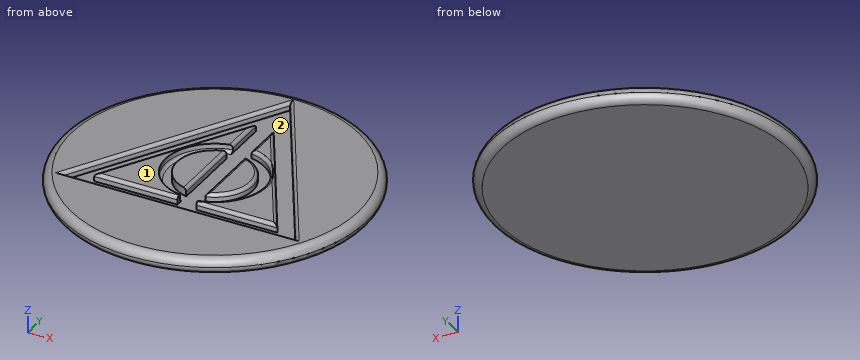
from build123d import *

# Parameters (mm, degrees)
F0_R         = 47.5
F1_DEPTH     = 5
F3_DEPTH     = 2.5
F4_R         = 15.4938561144
F4_R_2       = 11.9238234347
F5_DEPTH     = 2.5
F7_DEPTH     = 2.5
F8_R         = 2.49999
F9_T1_DEPTH  = 79.5044599257
F9_T6_ANGLE  = 178.5086872517
F9_T8_DEPTH  = 27.9406148573
F9_T10_DEPTH = 28.2323532374
F9_T12_DEPTH = 17.7111990238
F9_T14_DEPTH = 18.2220956401
F9_T16_DEPTH = 31.2335819135
F9_T18_DEPTH = 30.5369030224
F9_T20_DEPTH = 56.4226854656
F9_T22_DEPTH = 57.113596888
F9_T25_ANGLE = 172.3459061433
F9_T27_ANGLE = 174.2406786555
F9_T31_DEPTH = 79.5044599257
F9_T37_DEPTH = 79.5044599257
F9_T44_DEPTH = 79.5044599257
F9_T48_DEPTH = 79.5044599257


# Not quite as in the source:
# - a fillet or chamfer that OpenCascade refuses, or shapes differently, is made with other operations: its cross-section is extruded or revolved along the edge and cut away or added
# - a fillet or chamfer is up to 0.001 mm smaller than in the source, because OpenCascade refuses the exact size


with BuildPart() as f1:
    # F0 (on Top) → F1 (new body)
    with BuildSketch(Plane.XY):
        Circle(F0_R)
    extrude(amount=F1_DEPTH)

    # F2 (on face) → F3 (cut)
    with BuildSketch(Plane.XY.offset(5)):
        Polygon((-37.336189985, -21.3615019839), (37.1676983736, -21.6533380156), (0.1684916114, 43.0148399995), align=None)
        Polygon((-28.924478218, -16.5488310158), (0.1305310463, 33.3237484359), (28.7939471716, -16.77491742), align=None, mode=Mode.SUBTRACT)
    extrude(amount=-F3_DEPTH, mode=Mode.SUBTRACT)

    # F4 (on face) → F5 (cut)
    with BuildSketch(Plane.XY.offset(5)):
        Circle(F4_R)
        Circle(F4_R_2, mode=Mode.SUBTRACT)
    extrude(amount=-F5_DEPTH, mode=Mode.SUBTRACT)

    # F6 (on face) → F7 (cut)
    with BuildSketch(Plane.XY.offset(5)):
        with BuildLine():
            Line((3.2572400577, 27.8588049238), (0.1305310463, 33.3237484359))
            Line((0.1305310463, 33.3237484359), (-2.6910975575, 28.4804563395))
            Line((-2.6910975575, 28.4804563395), (-2.6910975575, 15.2583606993))
            ThreePointArc((-2.6910975575, 15.2583606993), (0.2884371491, 15.491171076), (3.2572400577, 15.1476059))
            Line((3.2572400577, 15.1476059), (3.2572400577, 27.8588049238))
        make_face()
        with BuildLine():
            ThreePointArc((3.2572400577, 15.1476059), (0.2884371491, 15.491171076), (-2.6910975575, 15.2583606993))
            Line((-2.6910975575, 15.2583606993), (-2.6910975575, -15.2583606993))
            ThreePointArc((-2.6910975575, -15.2583606993), (0.2884371491, -15.491171076), (3.2572400577, -15.1476059))
            Line((3.2572400577, -15.1476059), (3.2572400577, 15.1476059))
        make_face()
        with BuildLine():
            ThreePointArc((3.2572400577, -15.1476059), (0.2884371491, -15.491171076), (-2.6910975575, -15.2583606993))
            Line((-2.6910975575, -15.2583606993), (-2.6910975575, -16.6515886823))
            Line((-2.6910975575, -16.6515886823), (3.2572400577, -16.6748886641))
            Line((3.2572400577, -16.6748886641), (3.2572400577, -15.1476059))
        make_face()
    extrude(amount=-F7_DEPTH, mode=Mode.SUBTRACT)

    # F8 (radius 2.5 in the source; OpenCascade refuses exactly that, so slightly less here)
    f8_edges = [f1.edges().sort_by_distance(p)[0] for p in [
        (-47.5, 0, 5),
        (-47.5, 0, 0),
    ]]
    fillet(f8_edges, radius=F8_R)

    # F9: fillet of radius 1 on 14 edges, made by hand

    # F9_s2 → F9_t1 (join)
    with BuildSketch(Plane(origin=(-39.7519250003, 0.155710585, 0), x_dir=(0, 0, 1), z_dir=(0.9999923284, -0.0039170277, 0))):
        with BuildLine():
            ThreePointArc((3.5, 21.507584997), (2.7928932188, 21.2146917781), (2.5, 20.507584997))
            Line((2.5, 20.507584997), (2.5, 21.507584997))
            Line((2.5, 21.507584997), (3.5, 21.507584997))
        make_face()
    extrude(amount=F9_T1_DEPTH)


with BuildPart() as f9_tool4:
    # F9_s5 → F9_t6 (revolve)
    with BuildSketch(Plane(origin=(0, 0, 0), x_dir=(0, 0, 1), z_dir=(0.999915317, 0.0130137915, 0))):
        with BuildLine():
            ThreePointArc((2.5, -14.4938561144), (2.7928932188, -15.2009628956), (3.5, -15.4938561144))
            Line((3.5, -15.4938561144), (2.5, -15.4938561144))
            Line((2.5, -15.4938561144), (2.5, -14.4938561144))
        make_face()
    revolve(axis=Axis((0, 0, 2.5), (0, 0, 1)), revolution_arc=F9_T6_ANGLE)

    split(bisect_by=Plane.YZ.offset(-2.6910975575), keep=Keep.BOTTOM)


with BuildPart() as f1_1:
    add(f1.part)

    # F9_t3: union F9_tool4
    add(f9_tool4.part)

    # F9_s9 → F9_t8 (cut)
    with BuildSketch(Plane.XZ.offset(-13.9703074287)):
        with BuildLine():
            ThreePointArc((4.2572400577, 5), (3.5501332765, 4.7071067812), (3.2572400577, 4))
            Line((3.2572400577, 4), (3.2572400577, 5))
            Line((3.2572400577, 5), (4.2572400577, 5))
        make_face()
    extrude(amount=F9_T8_DEPTH, mode=Mode.SUBTRACT)

    # F9_s11 → F9_t10 (cut)
    with BuildSketch(Plane.XZ.offset(-14.1161766187)):
        with BuildLine():
            ThreePointArc((-2.6910975575, 4), (-2.9839907764, 4.7071067812), (-3.6910975575, 5))
            Line((-3.6910975575, 5), (-2.6910975575, 5))
            Line((-2.6910975575, 5), (-2.6910975575, 4))
        make_face()
    extrude(amount=F9_T10_DEPTH, mode=Mode.SUBTRACT)

    # F9_s13 → F9_t12 (cut)
    with BuildSketch(Plane.XZ.offset(-30.3588049238)):
        with BuildLine():
            ThreePointArc((4.2572400577, 5), (3.5501332765, 4.7071067812), (3.2572400577, 4))
            Line((3.2572400577, 4), (3.2572400577, 5))
            Line((3.2572400577, 5), (4.2572400577, 5))
        make_face()
    extrude(amount=F9_T12_DEPTH, mode=Mode.SUBTRACT)

    # F9_s15 → F9_t14 (cut)
    with BuildSketch(Plane.XZ.offset(-30.9804563395)):
        with BuildLine():
            ThreePointArc((-3.6910975575, 5), (-2.9839907764, 4.7071067812), (-2.6910975575, 4))
            Line((-2.6910975575, 4), (-2.6910975575, 5))
            Line((-2.6910975575, 5), (-3.6910975575, 5))
        make_face()
    extrude(amount=F9_T14_DEPTH, mode=Mode.SUBTRACT)

    # F9_s17 → F9_t16 (cut)
    with BuildSketch(Plane(origin=(-0.1258512133, 0.0004929665, 0), x_dir=(0, 0, 1), z_dir=(-0.9999923284, 0.0039170277, 0))):
        with BuildLine():
            ThreePointArc((5, -15.6620020419), (4.7071067812, -16.369108823), (4, -16.6620020419))
            Line((4, -16.6620020419), (5, -16.6620020419))
            Line((5, -16.6620020419), (5, -15.6620020419))
        make_face()
    extrude(amount=F9_T16_DEPTH, mode=Mode.SUBTRACT)

    # F9_s19 → F9_t18 (cut)
    with BuildSketch(Plane(origin=(31.3591935158, -0.1228357713, 0), x_dir=(0, 0, 1), z_dir=(-0.9999923284, 0.0039170277, 0))):
        with BuildLine():
            ThreePointArc((5, -15.6620020419), (4.7071067812, -16.369108823), (4, -16.6620020419))
            Line((4, -16.6620020419), (5, -16.6620020419))
            Line((5, -16.6620020419), (5, -15.6620020419))
        make_face()
    extrude(amount=F9_T18_DEPTH, mode=Mode.SUBTRACT)

    # F9_s21 → F9_t20 (cut)
    with BuildSketch(Plane(origin=(-12.4465088481, 21.7543326005, 0), x_dir=(0, 0, 1), z_dir=(0.4966039187, -0.8679772738, 0))):
        with BuildLine():
            ThreePointArc((4, -16.6620020419), (4.7071067812, -16.369108823), (5, -15.6620020419))
            Line((5, -15.6620020419), (5, -16.6620020419))
            Line((5, -16.6620020419), (4, -16.6620020419))
        make_face()
    extrude(amount=F9_T20_DEPTH, mode=Mode.SUBTRACT)

    # F9_s23 → F9_t22 (cut)
    with BuildSketch(Plane(origin=(-15.7859756564, -27.0964403413, 0), x_dir=(0, 0, 1), z_dir=(0.5033884097, 0.8640602462, 0))):
        with BuildLine():
            ThreePointArc((5, -15.6620020419), (4.7071067812, -16.369108823), (4, -16.6620020419))
            Line((4, -16.6620020419), (5, -16.6620020419))
            Line((5, -16.6620020419), (5, -15.6620020419))
        make_face()
    extrude(amount=F9_T22_DEPTH, mode=Mode.SUBTRACT)

    # F9_s24 → F9_t25 (revolve, cut)
    with BuildSketch(Plane(origin=(0, 0, 0), x_dir=(0, 0, 1), z_dir=(-0.997770072, 0.0667449131, 0))):
        with BuildLine():
            ThreePointArc((4, 11.9238234347), (4.7071067812, 11.6309302159), (5, 10.9238234347))
            Line((5, 10.9238234347), (5, 11.9238234347))
            Line((5, 11.9238234347), (4, 11.9238234347))
        make_face()
    revolve(axis=Axis((0, 0, 5), (0, 0, -1)), revolution_arc=F9_T25_ANGLE, mode=Mode.SUBTRACT)

    # F9_s26 → F9_t27 (revolve, cut)
    with BuildSketch(Plane(origin=(0, 0, 0), x_dir=(0, 0, 1), z_dir=(-0.9987372542, 0.0502384033, 0))):
        with BuildLine():
            ThreePointArc((5, 16.4938561144), (4.7071067812, 15.7867493333), (4, 15.4938561144))
            Line((4, 15.4938561144), (5, 15.4938561144))
            Line((5, 15.4938561144), (5, 16.4938561144))
        make_face()
    revolve(axis=Axis((0, 0, 5), (0, 0, -1)), revolution_arc=F9_T27_ANGLE, mode=Mode.SUBTRACT)


with BuildPart() as f9_tool29:
    # F9_s30 → F9_t31 (new body)
    with BuildSketch(Plane(origin=(20.0108118224, 34.3483216071, 0), x_dir=(0, 0, 1), z_dir=(-0.5033884097, -0.8640602462, 0))):
        with BuildLine():
            ThreePointArc((5, 22.507584997), (4.7071067812, 21.8004782158), (4, 21.507584997))
            Line((4, 21.507584997), (5, 21.507584997))
            Line((5, 21.507584997), (5, 22.507584997))
        make_face()
    extrude(amount=F9_T31_DEPTH)

    split(bisect_by=Plane(origin=(18.6680949925, 10.680750992, 0), x_dir=(0, 0, 1), z_dir=(-0.8679772738, -0.4966039187, 0)), keep=Keep.TOP)

    split(bisect_by=Plane(origin=(-0.0842458057, -21.5074199997, 0), x_dir=(0, 0, 1), z_dir=(0.0039170277, 0.9999923284, 0)), keep=Keep.TOP)


with BuildPart() as f1_2:
    add(f1_1.part)

    # F9_t28: cut F9_tool29
    add(f9_tool29.part, mode=Mode.SUBTRACT)


with BuildPart() as f9_tool35:
    # F9_s36 → F9_t37 (new body)
    with BuildSketch(Plane(origin=(19.7411131779, -34.5040321921, 0), x_dir=(0, 0, 1), z_dir=(-0.4966039187, 0.8679772738, 0))):
        with BuildLine():
            ThreePointArc((5, 22.507584997), (4.7071067812, 21.8004782158), (4, 21.507584997))
            Line((4, 21.507584997), (5, 21.507584997))
            Line((5, 21.507584997), (5, 22.507584997))
        make_face()
    extrude(amount=F9_T37_DEPTH)

    split(bisect_by=Plane(origin=(-18.5838491868, 10.8266690078, 0), x_dir=(0, 0, 1), z_dir=(0.8640602462, -0.5033884097, 0)), keep=Keep.TOP)

    split(bisect_by=Plane(origin=(-0.0842458057, -21.5074199997, 0), x_dir=(0, 0, 1), z_dir=(0.0039170277, 0.9999923284, 0)), keep=Keep.TOP)


with BuildPart() as f1_3:
    add(f1_2.part)

    # F9_t34: cut F9_tool35
    add(f9_tool35.part, mode=Mode.SUBTRACT)


with BuildPart() as f9_tool42:
    # F9_s43 → F9_t44 (new body)
    with BuildSketch(Plane(origin=(20.0108118224, 34.3483216071, 0), x_dir=(0, 0, 1), z_dir=(-0.5033884097, -0.8640602462, 0))):
        with BuildLine():
            ThreePointArc((5, 22.507584997), (4.7071067812, 21.8004782158), (4, 21.507584997))
            Line((4, 21.507584997), (5, 21.507584997))
            Line((5, 21.507584997), (5, 22.507584997))
        make_face()
    extrude(amount=F9_T44_DEPTH)

    split(bisect_by=Plane(origin=(18.6680949925, 10.680750992, 0), x_dir=(0, 0, 1), z_dir=(0.8679772738, 0.4966039187, 0)), keep=Keep.TOP)


with BuildPart() as f9_tool46:
    # F9_s47 → F9_t48 (new body)
    with BuildSketch(Plane(origin=(19.7411131779, -34.5040321921, 0), x_dir=(0, 0, 1), z_dir=(-0.4966039187, 0.8679772738, 0))):
        with BuildLine():
            ThreePointArc((5, 22.507584997), (4.7071067812, 21.8004782158), (4, 21.507584997))
            Line((4, 21.507584997), (5, 21.507584997))
            Line((5, 21.507584997), (5, 22.507584997))
        make_face()
    extrude(amount=F9_T48_DEPTH)

    split(bisect_by=Plane(origin=(-18.5838491868, 10.8266690078, 0), x_dir=(0, 0, 1), z_dir=(-0.8640602462, 0.5033884097, 0)), keep=Keep.TOP)


with BuildPart() as f9_tool42_1:
    add(f9_tool42.part)

    # F9_t50: intersect F9_tool46
    add(f9_tool46.part, mode=Mode.INTERSECT)


with BuildPart() as f1_4:
    add(f1_3.part)

    # F9_t40: cut F9_tool42
    add(f9_tool42_1.part, mode=Mode.SUBTRACT)


solid = f1_4.part
Can you work these out from the model? Positions are in its coordinate system, mm. Face numbers are marked on the shaded views. Give positions to 0.01 mm unless a question says otherwise; leave off trailing zeros. Write each loop counter-clockwise with the first axis right and the second up, starting at its lowest first coordinate (ties: lowest second). Pieces come first, ordered by that corner, then holes. Notation, with made-up numbers: M 72,-33.75 L 111,-33.75 A14 cw 111,-24.75 Z; hole C -11,83 d4. An arc over 180 degrees is marked long. Answer in a Markdown table with one row per item. Add a question column.
Item 1: For pin 1 Ø1.2 at (y, z) = (-16, 3.5) entering from +X; pin 2 Ø0.5 at (y, z) = (20.5, 3.5) entering from +X; pin 3 Ø1 at (x, z) = (-25.5, 1) entering from -Y, each with a flat end and sliding along its axis, tell me the tip position at first contact or that it passes through.
Item 2: We'd pull the mould along X, two halves only. Please class the marked faces 1 and 2: released by +X, released by -X, zero draft, split by the parting line, or undercut.
Item 3: Imagine slicing it at A-A, the plane z = 1.3. Write out the boundary of the cut face in (x, y).
Item 4: Please list where these lines run through material, in increasing order: L1, parallel to Y at x = -14, z = 3.65; L2, parallel to X at y = 9, z = 4.35; L3, parallel to Y at x = 13.5, z = 3.1.
Evaluation:
| question | item | result |
|---|---|---|
| 1 | pin 1 | stops at x = 44.8 |
| 1 | pin 2 | stops at x = 42.78 |
| 1 | pin 3 | stops at y = -39.97 |
| 2 | face 1 | zero draft |
| 2 | face 2 | undercut |
| 3 | outline | C 0,0 d94.39 |
| 4 | L1 | y = -45.1 to -21.45, -16.61 to -6.64, 6.64 to 9.07, 18.69 to 45.1 |
| 4 | L2 | x = -45.81 to -19.72, -13.97 to -12.61, -7.82 to -2.75, 3.32 to 7.72, 12.69 to 13.97, 19.7 to 45.81 |
| 4 | L3 | y = -45.46 to -21.48, -16.72 to -7.6, 7.6 to 9.96, 19.71 to 45.46 |
